For this review, take the finished solid that the model builds, in its own axes (mm). A direction names the side the tool comes from. Coordinates: 2 decimals unless noted, no trailing zeros. Write each loop counter-clockwise with the first axis right and the second up, starting at its lowest first coordinate (ties: lowest second). Pieces come first, ordered by that corner, then holes.
```python
from build123d import *

# Parameters (mm, degrees)
BOSS_EXTRUDE1_DEPTH = 8
SKETCH2_R           = 2.032
CUT_EXTRUDE1_DEPTH  = 14.144
BOSS_EXTRUDE2_DEPTH = 24
BOSS_EXTRUDE3_DEPTH = 8
BOSS_EXTRUDE4_DEPTH = 1.27
CUT_EXTRUDE2_DEPTH  = 1.27
MIRROR2_DEPTH       = 40
MIRROR2_START       = 32
MIRROR2_2_DEPTH     = 8
MIRROR2_3_OUTLINE_R = 2.032
MIRROR2_3_DEPTH     = 8
MIRROR2_START_2     = -1.27
MIRROR2_4_DEPTH     = 1.27


# Read off the part's stored shape, not the designer's step: Mirror2
with BuildPart() as part:
    # Sketch1 → Boss-Extrude1 (new body)
    with BuildSketch(Plane.XY):
        Polygon((-21, 16.936), (-21, 0), (0, 0), (0, 21), (-16.936, 21), align=None)
    boss_extrude1 = extrude(amount=BOSS_EXTRUDE1_DEPTH)

    # Sketch2 → Cut-Extrude1 (cut)
    with BuildSketch(Plane.XY.offset(8)):
        with Locations((-16.094318041, 16.094318041)):
            Circle(SKETCH2_R)
    cut_extrude1 = extrude(amount=-CUT_EXTRUDE1_DEPTH, mode=Mode.SUBTRACT)

    # Sketch4 → Boss-Extrude2 (add)
    with BuildSketch(Plane.XY.offset(8)):
        Polygon((0, 0), (-16.51, 0), (-16.51, 11.938), (-11.938, 16.51), (0, 16.51), align=None)
    boss_extrude2 = extrude(amount=BOSS_EXTRUDE2_DEPTH)

    # Sketch5 → Boss-Extrude3 (add)
    with BuildSketch(Plane.XY.offset(32)):
        Polygon((0, 0), (0, 21), (-16.936, 21), (-21, 16.936), (-21, 0), align=None)
    boss_extrude3 = extrude(amount=BOSS_EXTRUDE3_DEPTH)

    # Sketch6 → Boss-Extrude4 (add)
    with BuildSketch(Plane(origin=(0, 0, 0), x_dir=(-1, 0, 0), z_dir=(0, 0, -1))):
        with BuildLine():
            Line((0, 6.35), (0, 0))
            Line((0, 0), (6.35, 0))
            ThreePointArc((6.35, 0), (4.490128061, 4.490128061), (0, 6.35))
        make_face()
    boss_extrude4 = extrude(amount=BOSS_EXTRUDE4_DEPTH)

    # Sketch7 → Cut-Extrude2 (cut)
    with BuildSketch(Plane(origin=(0, 0, -1.27), x_dir=(-1, 0, 0), z_dir=(0, 0, -1))):
        with BuildLine():
            Line((0, 5.08), (0, 0))
            Line((0, 0), (5.08, 0))
            ThreePointArc((5.08, 0), (3.592102448, 3.592102448), (0, 5.08))
        make_face()
    cut_extrude2 = extrude(amount=-CUT_EXTRUDE2_DEPTH, mode=Mode.SUBTRACT)

    # Mirror1: Boss-Extrude1, Cut-Extrude1, Boss-Extrude2, Boss-Extrude3, Boss-Extrude4, Cut-Extrude2 across Right Plane
    add(boss_extrude1.mirror(Plane(origin=(0, 0, 0), x_dir=(0, 0, -1), z_dir=(1, 0, 0))))
    add(cut_extrude1.mirror(Plane(origin=(0, 0, 0), x_dir=(0, 0, -1), z_dir=(1, 0, 0))), mode=Mode.SUBTRACT)
    add(boss_extrude2.mirror(Plane(origin=(0, 0, 0), x_dir=(0, 0, -1), z_dir=(1, 0, 0))))
    add(boss_extrude3.mirror(Plane(origin=(0, 0, 0), x_dir=(0, 0, -1), z_dir=(1, 0, 0))))
    add(boss_extrude4.mirror(Plane(origin=(0, 0, 0), x_dir=(0, 0, -1), z_dir=(1, 0, 0))))
    add(cut_extrude2.mirror(Plane(origin=(0, 0, 0), x_dir=(0, 0, -1), z_dir=(1, 0, 0))), mode=Mode.SUBTRACT)

    # Mirror2 outline → Mirror2 (add)
    with BuildSketch(Plane.XY):
        Polygon((-16.51, 0), (-16.51, -11.938), (-11.938, -16.51), (11.938, -16.51), (16.51, -11.938), (16.51, 0), align=None)
    extrude(amount=MIRROR2_DEPTH)

    # Mirror2 2 outline → Mirror2 2 (add)
    with BuildSketch(Plane.XY.offset(MIRROR2_START)):
        Polygon((-21, 0), (-21, -16.936), (-16.936, -21), (16.936, -21), (21, -16.936), (21, 0), (16.51, 0), (16.51, -11.938), (11.938, -16.51), (-11.938, -16.51), (-16.51, -11.938), (-16.51, 0), align=None)
    extrude(amount=MIRROR2_2_DEPTH)

    # Mirror2 3 outline → Mirror2 3 (add)
    with BuildSketch(Plane.XY):
        Polygon((-21, 0), (-21, -16.936), (-16.936, -21), (16.936, -21), (21, -16.936), (21, 0), (16.51, 0), (16.51, -11.938), (11.938, -16.51), (-11.938, -16.51), (-16.51, -11.938), (-16.51, 0), align=None)
        with Locations((-16.094318041, -16.094318041)):
            Circle(MIRROR2_3_OUTLINE_R, mode=Mode.SUBTRACT)
        with Locations((16.094318041, -16.094318041)):
            Circle(MIRROR2_3_OUTLINE_R, mode=Mode.SUBTRACT)
    extrude(amount=MIRROR2_3_DEPTH)

    # Mirror2 4 outline → Mirror2 4 (add)
    with BuildSketch(Plane.XY.offset(MIRROR2_START_2)):
        with BuildLine():
            Line((-5.08, 0), (-6.35, 0))
            ThreePointArc((-6.35, 0), (0, -6.35), (6.35, 0))
            Line((6.35, 0), (5.08, 0))
            ThreePointArc((5.08, 0), (0, -5.08), (-5.08, 0))
        make_face()
    extrude(amount=MIRROR2_4_DEPTH)


solid = part.part
```
Q1. Tool access review of faces 5 (the flat face through (0, 19, 8)), 6 (the flat face through (-5, 5, 0)), 7 (the flat face through (16.51, 0, 20)), 8 (the flat face through (-16.51, 0, 20)): name each direction out of +Z, -Z, +X, -X, +Y, -Y from which nothing blocks a thin tool from reaching the whole face with its end or side.
Ans:
face 5: none
face 6: -Z
face 7: +X, +Y, -Y
face 8: -X, +Y, -Y
Q2. Draft analysis for pull direction X (two halves, no side actions). For faces 1 (the flat face through (0, 0, 0)), 2 (the flat face through (0, 21, 36)), 3 (the cylindrical face through (-17.59, 17.47, 4.06)), 4 (the flat face through (-18.94, 18.996, 3.944)), state which applies: +X half, -X half, draft (parallel to the pull), parting line (faces both ways), or undercut.
Ans:
face 1: undercut
face 2: draft
face 3: undercut
face 4: -X half
Q3. For probe 1 along Z at (x, y) = (19, -7); probe 2 along X at (y, z) = (5, 31.5), list the stretches that pass through material, from the lowest coordinate up.
Ans:
probe 1: z = 0 to 8, 32 to 40
probe 2: x = -16.51 to 16.51
Q4. Add section A-A (x = 11). State the section outline as (y, z) points.
Ans:
outline: (-21, 0) - (21, 0) - (21, 8) - (16.51, 8) - (16.51, 32) - (21, 32) - (21, 40) - (-21, 40) - (-21, 32) - (-16.51, 32) - (-16.51, 8) - (-21, 8) - close
Q5. Add section D-D (z = 36). State the section outline as (x, y) points.
Ans:
outline: (-21, -16.94) - (-16.94, -21) - (16.94, -21) - (21, -16.94) - (21, 16.94) - (16.94, 21) - (-16.94, 21) - (-21, 16.94) - close
Q6. Add section B-B (z = 28). State the section outline as (x, y) points.
Ans:
outline: (-16.51, -11.94) - (-11.94, -16.51) - (11.94, -16.51) - (16.51, -11.94) - (16.51, 11.94) - (11.94, 16.51) - (-11.94, 16.51) - (-16.51, 11.94) - close
Q7. Clearance check with flat-ended pins moving along their axes: pin 1 Ø3 at (x, z) = (2.5, 16.5) entering from -Y; pin 2 Ø3 at (x, z) = (-8, 26) entering from +Y; pin 3 Ø6.5 at (x, y) = (-16.09, 16.09) entering from -Z. State where each tip first meets the part, or that it passes through.
Ans:
pin 1: stops at y = -16.51
pin 2: stops at y = 16.51
pin 3: stops at z = 0
